Answer from the drawing. Dimensions are ordinates in mm from the lowest x, y and z of the part. Round coordinates to 2 decimals unless told otherwise and drop trailing zeros. Loops run counter-clockwise (first coordinate to the right, second up) from the corner with the lowest first, then second, coordinate; pieces in that order, holes last. Notation, with made-up numbers: (65.5, 16) - (74.5, 16) arc R23 ccw to (74.5, 34) - close; hole circle Ø1 at (46, 34.25). An arc over 180 degrees is marked (long way). Answer as CSV lines item,"result". Start each with the question number.
Q1. Straight lines are drawn through the part: L1, parallel to Y at x = 1.9, z = 7.5; L2, parallel to Z at x = 2.5, y = 7.5; L3, parallel to X at y = 7.75, z = 13.5. For each, find the intervals that lie inside material, in ascending order. Write a range as [from, to].
Q2. Section D-D on x = 2.6 is taken. Write down the section's boundary in (y, z), then the cut area to 3 significant figures.
Q3. Section A-A on z = 7.5 is taken. Write down the section's boundary in (x, y).
Q4. This flat-tipped pin is pushed along its axis until it touches: pin 1 Ø1.1 at (x, z) = (2.5, 4.5) entering from +Y. Where does it stop, or does it pass through?
Q5. The mould has two halves that part along Y. Classify the marked faces 1, 2 and 3: +Y half, -Y half, draft (parallel to the pull), parting line (faces both ways), or undercut.
Q6. Section C-C on y = 9.25 is taken. Write down the section's boundary in (x, z).
Q7. Section B-B on y = 7.5 is taken. Write down the section's boundary in (x, z).
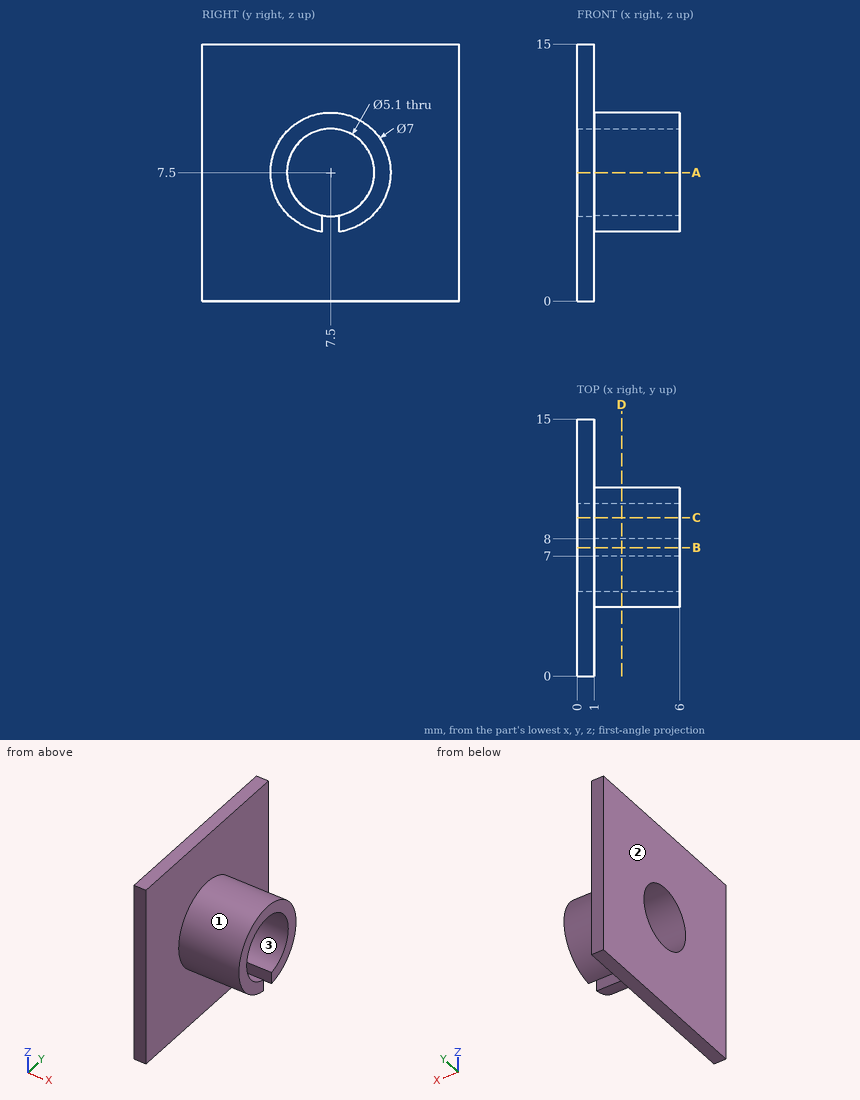
Findings:
1,L1,"y = [4, 4.95], [10.05, 11]"
1,L2,"z = [10.05, 11]"
1,L3,"x = [0, 1]"
2,outline,"(7, 4.04) - (7, 5) arc R2.55 cw (long way) to (8, 5) - (8, 4.04) arc R3.5 ccw (long way) to start"
2,area,"17.1 mm^2"
3,outline,"(0, 0) - (1, 0) - (1, 4) - (6, 4) - (6, 4.95) - (0, 4.95) - close; (0, 10.05) - (6, 10.05) - (6, 11) - (1, 11) - (1, 15) - (0, 15) - close"
4,pin 1,"stops at y = 10"
5,face 1,"parting line"
5,face 2,"draft"
5,face 3,"undercut"
6,outline,"(0, 0) - (1, 0) - (1, 4.47) - (6, 4.47) - (6, 5.65) - (0, 5.65) - close; (0, 9.35) - (6, 9.35) - (6, 10.53) - (1, 10.53) - (1, 15) - (0, 15) - close"
7,outline,"(0, 0) - (1, 0) - (1, 4.95) - (0, 4.95) - close; (0, 10.05) - (6, 10.05) - (6, 11) - (1, 11) - (1, 15) - (0, 15) - close"
